Source: CAD feature listing. Evaluate the final solid. Frame: model axes, mm. A direction names the side the tool comes from. Give positions to 0.01 mm unless a question says otherwise; leave off trailing zeros. Order: outer loops, then holes, each group sorted by start corner. A loop starts at its lowest first (then second) coordinate and runs counter-clockwise, first axis right, second up.
```python
from build123d import *

# Parameters (mm, degrees)
SKETCH1_W           = 3
SKETCH1_H           = 19
SKETCH1_R           = 1
SKETCH1_R_2         = 15.5
BOSS_EXTRUDE1_DEPTH = 3


with BuildPart() as part:
    # Sketch1 → Boss-Extrude1 (new body)
    with BuildSketch(Plane(origin=(0, 0, 0), x_dir=(1, 0, 0), z_dir=(0, 1, 0))):
        Polygon((33.333333333, 21.5), (0, 21.5), (0, 18.5), (-4, 18.5), (-4, -18.5), (0, -18.5), (0, -21.5), (33.333333333, -21.5), (33.333333333, -18.5), (73.333333333, -18.5), (73.333333333, -21.5), (106.666666667, -21.5), (106.666666667, -18.5), (146.666666667, -18.5), (146.666666667, -21.5), (180, -21.5), (180, 21.5), (146.666666667, 21.5), (146.666666667, 18.5), (106.666666667, 18.5), (106.666666667, 21.5), (73.333333333, 21.5), (73.333333333, 18.5), (33.333333333, 18.5), align=None)
        with Locations((1.5, 0)):
            Rectangle(SKETCH1_W, SKETCH1_H, mode=Mode.SUBTRACT)
        with Locations((74.375, -13)):
            Circle(SKETCH1_R, mode=Mode.SUBTRACT)
        with Locations((142.875, -13)):
            Circle(SKETCH1_R, mode=Mode.SUBTRACT)
        with Locations((23, 0)):
            Circle(SKETCH1_R_2, mode=Mode.SUBTRACT)
        with Locations((57.25, 0)):
            Circle(SKETCH1_R_2, mode=Mode.SUBTRACT)
        with Locations((74.375, 13)):
            Circle(SKETCH1_R, mode=Mode.SUBTRACT)
        with Locations((91.5, 0)):
            Circle(SKETCH1_R_2, mode=Mode.SUBTRACT)
        with Locations((125.75, 0)):
            Circle(SKETCH1_R_2, mode=Mode.SUBTRACT)
        with Locations((160, 0)):
            Circle(SKETCH1_R_2, mode=Mode.SUBTRACT)
        with Locations((142.875, 13)):
            Circle(SKETCH1_R, mode=Mode.SUBTRACT)
    extrude(amount=BOSS_EXTRUDE1_DEPTH)


solid = part.part
```
1) Section query B-B, the plane z = 0. Return the cut outline in (x, y), and give its area (3 significant figures).
Report:
outline: (-4, 0) - (0, 0) - (0, 3) - (-4, 3) - close; (3, 0) - (7.5, 0) - (7.5, 3) - (3, 3) - close; (38.5, 0) - (41.75, 0) - (41.75, 3) - (38.5, 3) - close; (72.75, 0) - (76, 0) - (76, 3) - (72.75, 3) - close; (107, 0) - (110.25, 0) - (110.25, 3) - (107, 3) - close; (141.25, 0) - (144.5, 0) - (144.5, 3) - (141.25, 3) - close; (175.5, 0) - (180, 0) - (180, 3) - (175.5, 3) - close
area: 78.0 mm2
2) Reachability of faces 4 (the flat face through (146.667, 1, 20)), 5 (the flat face through (1, 1, 9.5)), 6 (the flat face through (54, 1, -18.5)), 7 (the flat face through (66, 0, -15)) from +Z, -Z, +X, -X, +Y, -Y: full face, straight path, thin tool, end or side. Return the list, or none.
Report:
face 4: +Z, +Y, -Y
face 5: +Y, -Y
face 6: -Z, +Y, -Y
face 7: +Z, -Z, +X, -X, -Y
3) Section query C-C, the plane y = 1.25. Count the separate pieces of the cut face and the enclosed holes in it, and give its area (3 significant figures).
Report:
separate pieces: 1
enclosed holes: 10
area: 3,560 mm2
4) Section query A-A, the plane x = 160. Return the cut outline in (y, z).
Report:
outline: (0, -21.5) - (3, -21.5) - (3, -15.5) - (0, -15.5) - close; (0, 15.5) - (3, 15.5) - (3, 21.5) - (0, 21.5) - close
5) Section query D-D, the plane x = 125.75. Return the cut outline in (y, z), and give its area (3 significant figures).
Report:
outline: (0, -18.5) - (3, -18.5) - (3, -15.5) - (0, -15.5) - close; (0, 15.5) - (3, 15.5) - (3, 18.5) - (0, 18.5) - close
area: 18.0 mm2
6) Material intervals for L1, parallel to Z at x = 125.5, y = 2.9; L2, parallel to X at y = 1.2, z = 10.5; L3, parallel to Z at x = 160, y = 2.15, sorted ascending.
Report:
L1: z = -18.5 to -15.5, 15.5 to 18.5
L2: x = -4 to 11.6, 34.4 to 45.85, 68.65 to 80.1, 102.9 to 114.35, 137.15 to 148.6, 171.4 to 180
L3: z = -21.5 to -15.5, 15.5 to 21.5
7) Pin query (flat end, axial travel): pin 1 (0.9 mm diameter, centred on y = 2, z = -20, fed in from -X); pin 2 (1 mm diameter, centred on x = 34.5, y = 1.5, fed in from -Z). Return the tip coordinate at first contact, or that it passes through.
Report:
pin 1: stops at x = 0
pin 2: stops at z = -18.5
8) Draft query along Z for faces 1 (the flat face through (17, 1, -21.5)), 2 (the cylindrical face through (144.515, 1.479, -0.682)), 3 (the flat face through (146.667, 1, -20)). Return one class per face: +Z half, -Z half, draft (parallel to the pull), parting line (faces both ways), or undercut.
Report:
face 1: -Z half
face 2: undercut
face 3: draft
